```python
from build123d import *

# Parameters (mm, degrees)
CUT_EXTRUDE1_DEPTH      = 23
CUT_EXTRUDE1_DEPTH_BACK = 23
CUT_EXTRUDE2_DEPTH      = 23
CUT_EXTRUDE2_DEPTH_BACK = 23
SKETCH3_W               = 26
SKETCH3_H               = 13.5
SKETCH4_W               = 23
SKETCH4_H               = 3.16
SKETCH5_W               = 2.5
SKETCH5_H               = 23


with BuildPart() as part:
    # Sketch1 → Revolve1 (revolve)
    with BuildSketch(Plane.XY, mode=Mode.PRIVATE) as revolve1_sk:
        with BuildLine():
            Line((0, 10.5), (0, 7))
            Line((0, 7), (1, 6))
            Line((1, 6), (31.8, 6))
            Line((31.8, 6), (31.8, 11.5))
            Line((31.8, 11.5), (13.5, 11.5))
            Line((13.5, 11.5), (13.5, 10.5))
            Line((13.5, 10.5), (11.5, 10.5))
            Line((11.5, 10.5), (11.5, 11.5))
            Line((11.5, 11.5), (8.274596669, 11.5))
            ThreePointArc((8.274596669, 11.5), (7.5, 10.5), (6.725403331, 11.5))
            Line((6.725403331, 11.5), (1, 11.5))
            Line((1, 11.5), (0, 10.5))
        make_face()
    revolve(revolve1_sk.sketch.rotate(Axis((31.8, 0, 0), (-1, 0, 0)), 270), axis=Axis((31.8, 0, 0), (-1, 0, 0)))

    # Sketch2 → Cut-Extrude1 (cut, two sides: drawn at the far end of the back side and taken through both)
    with BuildSketch(Plane.XY.offset(-CUT_EXTRUDE1_DEPTH_BACK)):
        with BuildLine():
            Line((15, 12.5), (15, 9.8))
            ThreePointArc((15, 9.8), (16.171572875, 6.971572875), (19, 5.8))
            Line((19, 5.8), (26, 5.8))
            ThreePointArc((26, 5.8), (31.8, 0), (26, -5.8))
            Line((26, -5.8), (19, -5.8))
            ThreePointArc((19, -5.8), (16.171572875, -6.971572875), (15, -9.8))
            Line((15, -9.8), (15, -12.5))
            Line((15, -12.5), (41, -12.5))
            Line((41, -12.5), (41, 12.5))
            Line((41, 12.5), (15, 12.5))
        make_face()
    extrude(amount=CUT_EXTRUDE1_DEPTH + CUT_EXTRUDE1_DEPTH_BACK, mode=Mode.SUBTRACT)

    # Sketch3 → Cut-Extrude2 (cut, two sides: drawn at the far end of the back side and taken through both)
    with BuildSketch(Plane(origin=(0, 0, 0), x_dir=(1, 0, 0), z_dir=(0, 1, 0)).offset(-CUT_EXTRUDE2_DEPTH_BACK)):
        with Locations((28, 0)):
            Rectangle(SKETCH3_W, SKETCH3_H)
    extrude(amount=CUT_EXTRUDE2_DEPTH + CUT_EXTRUDE2_DEPTH_BACK, mode=Mode.SUBTRACT)

    # Sketch4 → Cut-Revolve1 (revolve, cut)
    with BuildSketch(Plane(origin=(26, 0, 0), x_dir=(0, 0, -1), z_dir=(1, 0, 0)), mode=Mode.PRIVATE) as cut_revolve1_sk:
        with Locations((0, 1.58)):
            Rectangle(SKETCH4_W, SKETCH4_H)
    revolve(cut_revolve1_sk.sketch.rotate(Axis((26, 0, -11.5), (0, 0, 1)), 90), axis=Axis((26, 0, -11.5), (0, 0, 1)), mode=Mode.SUBTRACT)

    # Sketch5 → Cut-Revolve2 (revolve, cut)
    with BuildSketch(Plane(origin=(7.5, 0, 0), x_dir=(0, 0, -1), z_dir=(1, 0, 0)), mode=Mode.PRIVATE) as cut_revolve2_sk:
        with Locations((1.25, 0)):
            Rectangle(SKETCH5_W, SKETCH5_H)
    revolve(cut_revolve2_sk.sketch.rotate(Axis((7.5, -11.5, 0), (0, 1, 0)), 180), axis=Axis((7.5, -11.5, 0), (0, 1, 0)), mode=Mode.SUBTRACT)


solid = part.part
```
Could you check a few things on this model? Use its own coordinates, in mm. A direction names the side the tool comes from. Round coordinates to 2 decimals unless told otherwise and drop trailing zeros. Write each loop counter-clockwise with the first axis right and the second up, starting at its lowest first coordinate (ties: lowest second). Pieces come first, ordered by that corner, then holes.
(1) If I drill on probe 1 along X at (y, z) = (8.5, 0); probe 2 along Y at (x, z) = (26, -8.5); probe 3 along Y at (x, z) = (20, -7), over which ranges is the centre line in solid material (lowest first)?
Findings below:
probe 1: x = 0 to 5, 10 to 15
probe 2: y = -5.8 to -3.16, 3.16 to 5.8
probe 3: y = -5.8 to 5.8
(2) Suppose I cut it at C-C on y = 0. State how many separate pieces and enclosed holes the cut face has, and give its area (3 significant figures).
Findings below:
separate pieces: 4
enclosed holes: 0
area: 256 mm2
(3) Suppose I cut it at B-B on z = 0. Write out the boundary of the cut face in (x, y).
Findings below:
outline: (0, -10.5) - (1, -11.5) - (5, -11.5) - (5, -6) - (1, -6) - (0, -7) - close; (0, 7) - (1, 6) - (5, 6) - (5, 11.5) - (1, 11.5) - (0, 10.5) - close; (10, -11.5) - (11.5, -11.5) - (11.5, -10.5) - (13.5, -10.5) - (13.5, -11.5) - (15, -11.5) - (15, -6) - (10, -6) - close; (10, 6) - (15, 6) - (15, 11.5) - (13.5, 11.5) - (13.5, 10.5) - (11.5, 10.5) - (11.5, 11.5) - (10, 11.5) - close
(4) Thinking about a two-plate mould opening in X: for faces 1 (the face through (31.8, 0.1, -8.6)), 2 (the face through (13.5, -10.2, 3.4)), 3 (the face through (0, -7, 2)), 4 (the face through (21, 0, -6.75)), which applies, +X half, -X half, draft (parallel to the pull), parting line (faces both ways), or undercut?
Findings below:
face 1: +X half
face 2: undercut
face 3: -X half
face 4: draft
(5) For pin 1 (8 mm diameter, centred on x = 4, y = 0.5, fed in from +Z); pin 2 (4 mm diameter, centred on x = 23, z = -8, fed in from +Y); pin 3 (4 mm diameter, centred on x = 7.5, z = 0, fed in from +Y); pin 4 (12 mm diameter, centred on x = 11.5, z = -7.5, fed in from +Y), each with a flat end and sliding along its axis, tell me the tip position at first contact or that it passes through.
Findings below:
pin 1: stops at z = 11.5
pin 2: stops at y = 5.8
pin 3: passes through
pin 4: stops at y = 11.4
(6) Which directions (+Z, -Z, +X, -X, +Y, -Y) give clear straight access to the entire face, cutting with the end or side of a thin tool? Please do faces 5 (the face through (31.8, 0.1, 8.6)), 6 (the face through (12.5, 3.2, 10)), 7 (the face through (15, -3, 6)).
Findings below:
face 5: +Z, -Z, +X
face 6: none
face 7: +X, +Y, -Y
(7) Suppose I cut it at D-D on x = 13. Write out the boundary of the cut face in (y, z), and give its area (3 significant figures).
Findings below:
outline: circle Ø21 at (0, 0); hole circle Ø12 at (0, 0)
area: 233 mm2
(8) Suppose I cut it at A-A on x = 21.5. Write out the boundary of the cut face in (y, z), and give its area (3 significant figures).
Findings below:
outline: (-5.8, -9.93) arc R11.5 ccw to (5.8, -9.93) - (5.8, -6.75) - (-5.8, -6.75) - close; (-5.8, 6.75) - (5.8, 6.75) - (5.8, 9.93) arc R11.5 ccw to (-5.8, 9.93) - close
area: 98.4 mm2
